from build123d import *

# Parameters (mm, degrees)
F0_W           = 64
F0_H           = 38
F0_W_2         = 38
F0_H_2         = 19
F1_DEPTH       = 2
F2_R           = 2
F4_D           = 3.2
F4_CBORE_D     = 6
F4_CBORE_DEPTH = 1


with BuildPart() as f1:
    # F0 (on Top) → F1 (new body)
    with BuildSketch(Plane.XY):
        with Locations((32, 19)):
            Rectangle(F0_W, F0_H)
        with Locations((30, 19)):
            Rectangle(F0_W_2, F0_H_2, mode=Mode.SUBTRACT)
    extrude(amount=F1_DEPTH)

    # F2
    f2_edges = [f1.edges().sort_by_distance(p)[0] for p in [
        (0, 38, 1),
        (0, 0, 1),
        (64, 0, 1),
        (64, 38, 1),
    ]]
    fillet(f2_edges, radius=F2_R)

    # F4 (through all)
    with Locations(Plane(origin=(0, 0, 0), x_dir=(1, 0, 0), z_dir=(0, 0, -1))):
        with Locations((2.5, -2.5), (2.5, -35.5), (61.5, -35.5), (61.5, -2.5)):
            CounterBoreHole(F4_D / 2, F4_CBORE_D / 2, F4_CBORE_DEPTH)


solid = f1.part
CAD build for the part. Positions are in the model's coordinates, mm. A direction names the side the tool comes from. Round coordinates to 2 decimals unless told otherwise and drop trailing zeros. Order: outer loops, then holes, each group sorted by start corner. A loop starts at its lowest first (then second) coordinate and runs counter-clockwise, first axis right, second up. Notation, with made-up numbers: (55.5, 24.25) -> (65.5, 24.25) arc R26 cw to (65.5, 59.25) -> close; hole circle Ø11 at (-20, -3.5). An arc over 180 degrees is marked (long way). Write item = value, one per line. Start each with the question number.
(1) Cut at B-B, the plane x = 42. List the corners of the cut face in (y, z), then the cut area to 3 significant figures.
(2) Pin check, flat tips, straight feed: P1, Ø2.5, axis at x = 2.5, y = 2.5, coming from the +Z side; P2, Ø5, axis at x = 48, y = 34, coming from the -Z side; P3, Ø5, axis at x = 2.5, y = 35.5, coming from the -Z side. Stop position of each tip, or through.
(3) Which spindle directions (+Z, -Z, +X, -X, +Y, -Y) get a long thin tool onto all of the face, cutting with end or side? Do faces 4 (the flat face through (30, 28.5, 1)), 5 (the cylindrical face through (0.57, 0.6, 1.51)), 6 (the flat face through (4, 34, 1)). Say none if no direction does.
(4) Cut at A-A, the plane z = 1.45. List the corners of the cut face in (x, y), then the cut area to 3 significant figures.
(5) Pull direction Y, two halves, no side cores. Call faces 1 (the flat face through (64, 19, 1)), 2 (the flat face through (49, 19, 1)), 3 (the cylindrical face through (63.4, 37.43, 1.51)): released by +Y, released by -Y, zero draft, split by the parting line, or undercut.
(6) Cut at C-C, the plane y = 23. List the corners of the cut face in (x, z), then the cut area to 3 significant figures.
(7) Probe line 1 (Y direction, x = 61.5, z = 1.85); line 2 (X direction, y = 35.5, z = 1.3); line 3 (X direction, y = 11.5, z = 0.65). List the from-to ranges inside material, lowest first. Write a range as [from, to].
Model answer:
q1.outline = (0, 0) -> (9.5, 0) -> (9.5, 2) -> (0, 2) -> close; (28.5, 0) -> (38, 0) -> (38, 2) -> (28.5, 2) -> close
q1.area = 38.0 mm2
q2.P1 = through
q2.P2 = 0
q2.P3 = 1
q3.face_4 = +Z, -Z
q3.face_5 = +Z, -Z, -X, -Y
q3.face_6 = -Z
q4.outline = (0, 2) arc R2 ccw to (2, 0) -> (62, 0) arc R2 ccw to (64, 2) -> (64, 36) arc R2 ccw to (62, 38) -> (2, 38) arc R2 ccw to (0, 36) -> close; hole circle Ø3.2 at (2.5, 2.5); hole circle Ø3.2 at (2.5, 35.5); hole (11, 9.5) -> (49, 9.5) -> (49, 28.5) -> (11, 28.5) -> close; hole circle Ø3.2 at (61.5, 2.5); hole circle Ø3.2 at (61.5, 35.5)
q4.area = 1,670 mm2
q5.face_1 = zero draft
q5.face_2 = undercut
q5.face_3 = released by +Y
q6.outline = (0, 0) -> (11, 0) -> (11, 2) -> (0, 2) -> close; (49, 0) -> (64, 0) -> (64, 2) -> (49, 2) -> close
q6.area = 52.0 mm2
q7.line_1 = [0, 0.9], [4.1, 33.9], [37.1, 38]
q7.line_2 = [0, 0.9], [4.1, 59.9], [63.1, 64]
q7.line_3 = [0, 11], [49, 64]
